Autodesk Inventor part; units mm, degrees
ref_plane "YZ Plane" through (0, 0, 0) normal (1, 0, 0) x (0, 1, 0)
ref_plane "XZ Plane" through (0, 0, 0) normal (0, 1, 0) x (-1, 0, 0)
ref_plane "XY Plane" through (0, 0, 0) normal (0, 0, 1) x (1, 0, 0)
sketch "Sketch1" plane through (0, 0, 0) normal (0, 0, 1) x (1, 0, 0)
  line L0 (-12.2998, 27.0657) -> (12.7002, 27.0657)
  line L1 (12.7002, 27.0657) -> (12.7002, -22.9343)
  line L2 (12.7002, -22.9343) -> (-12.2998, -22.9343)
  line L3 (-12.2998, -22.9343) -> (-12.2998, 27.0657)
  circle A0 centre (0, -20.3589) radius 1
  line L4 (-0.9186, 24.8477) -> (1.0814, 24.8477)
  line L5 (1.0814, 24.8477) -> (1.0814, 22.8477)
  line L6 (1.0814, 22.8477) -> (-0.9186, 22.8477)
  line L7 (-0.9186, 22.8477) -> (-0.9186, 24.8477)
  point P0 (0, 0)
  dimension "d0" = 25
  dimension "d1" = 50
  dimension "d2" = 2
  dimension "d3" = 2
  dimension "d4" = 2
extrude "Extrusion1" add sketch "Sketch1" along normal blind 2
properties part number "Lclamp1"
Source: CAD feature listing. Evaluate the final solid. Frame: model axes, mm. A direction names the side the tool comes from. Round coordinates to 2 decimals unless told otherwise and drop trailing zeros. Order: outer loops, then holes, each group sorted by start corner. A loop starts at its lowest first (then second) coordinate and runs counter-clockwise, first axis right, second up. Notation, with made-up numbers: (-33.5, -17.5) -> (8.5, -17.5) arc R9 cw to (8.5, -0.5) -> close; hole circle Ø7 at (76.25, 89). An arc over 180 degrees is marked (long way). One line per item, written item: value. Start each with the question number.
Q1. Draft query along X for faces 3 (the cylindrical face through (-0.13, -21.35, 0.99)), 4 (the flat face through (0, 27.066, 1)), 5 (the flat face through (12.7, 2, 1)). Return one class per face: pulls with the +X half, pulls with the -X half, needs draft (parallel to the pull), parting line crosses it, or undercut.
Q2. Access query for faces 1 (the flat face through (-12.3, 2, 1)), 2 (the flat face through (0, 24.848, 1)). Directions: +Z, -Z, +X, -X, +Y, -Y. A direction counts if a zero-diameter tool reaches every point of the face in a straight line with its end or side. Return the directions, or none.
Q3. Material intervals for probe 1 along Y at (x, z) = (0, 0.6); probe 2 along X at (y, z) = (-20, 0.4), sorted ascending.
Q4. Section query A-A (x = 0). Return the cut outline in (y, z).
Q5. Pin query (flat end, axial travel): pin 1 (3 mm diameter, centred on x = 0, y = -20.36, fed in from -Z). Return the tip coordinate at first contact, or that it passes through.
Findings below:
1. face 3: undercut
1. face 4: needs draft
1. face 5: pulls with the +X half
2. face 1: +Z, -Z, -X, +Y, -Y
2. face 2: +Z, -Z
3. probe 1: -22.93 to -21.36, -19.36 to 22.85, 24.85 to 27.07
3. probe 2: -12.3 to -0.93, 0.93 to 12.7
4. outline: (-22.93, 0) -> (-21.36, 0) -> (-21.36, 2) -> (-22.93, 2) -> close; (-19.36, 0) -> (22.85, 0) -> (22.85, 2) -> (-19.36, 2) -> close; (24.85, 0) -> (27.07, 0) -> (27.07, 2) -> (24.85, 2) -> close
5. pin 1: z = 0
